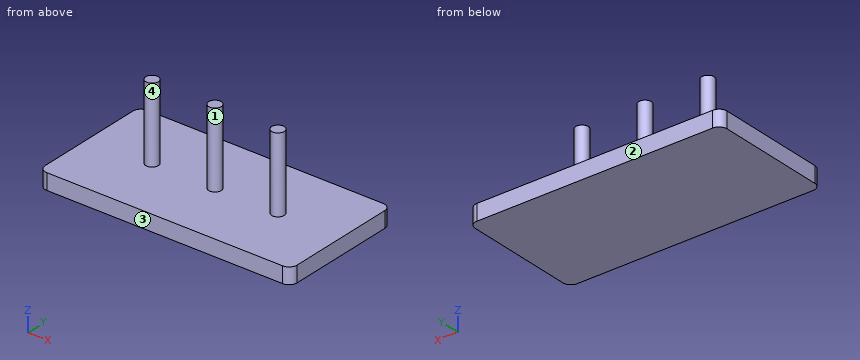
```python
from build123d import *

# Parameters (mm, degrees)
F0_W     = 400
F0_H     = 200
F1_DEPTH = 25.4
F2_R     = 10
F3_DEPTH = 120
F4_R     = 12.7


with BuildPart() as f1:
    # F0 (on Top) → F1 (new body)
    with BuildSketch(Plane.XY):
        Rectangle(F0_W, F0_H)
    extrude(amount=F1_DEPTH)

    # F2 (on face) → F3 (join)
    with BuildSketch(Plane.XY.offset(25.4)):
        Circle(F2_R)
        with Locations((100, 0)):
            Circle(F2_R)
        with Locations((-100, 0)):
            Circle(F2_R)
    extrude(amount=F3_DEPTH)

    # F4
    f4_edges = [f1.edges().sort_by_distance(p)[0] for p in [
        (200, -100, 12.7),
        (-200, -100, 12.7),
        (-200, 100, 12.7),
        (200, 100, 12.7),
    ]]
    fillet(f4_edges, radius=F4_R)


solid = f1.part
```
Work out the finished part from the listing and answer in its coordinate system (mm). Face numbers are marked on the shaded views. A direction names the side the tool comes from. Give positions to 0.01 mm unless a question says otherwise; leave off trailing zeros. Order: outer loops, then holes, each group sorted by start corner. A loop starts at its lowest first (then second) coordinate and runs counter-clockwise, first axis right, second up. Notation, with made-up numbers: M -11,45 L -5,45 A16 ccw -5,67 Z; hole C -25.75,89 d3. An arc over 180 degrees is marked long. Return JSON: item names as keys, results as strings.
1) Section D-D, the plane x = 62 is taken. Write down the section's boundary in (y, z), plus the area to 3 significant figures.
Resolved:
{"outline": "M -100,0 L 100,0 L 100,25.4 L -100,25.4 Z", "area": "5,080 mm^2"}
2) This flat-tipped pin is pushed along its axis until it touches: pin 1 (2 mm diameter, centred on x = -81.5, y = -56, fed in from +Z). Where does it stop, or does it pass through?
Resolved:
{"pin 1": "z = 25.4"}
3) Section C-C, the plane x = -100 is taken. Write down the section's boundary in (y, z), plus the area to 3 significant figures.
Resolved:
{"outline": "M -100,0 L 100,0 L 100,25.4 L 10,25.4 L 10,145.4 L -10,145.4 L -10,25.4 L -100,25.4 Z", "area": "7,480 mm^2"}
4) Straight lines are drawn through the part: line 1 along Z through (x, y) = (-171, -66); line 2 along X through (y, z) = (4, 28.5); line 3 along Y through (x, z) = (3, 39). For each, find the intervals that lie inside material, in ascending order. Write a range as [from, to].
Resolved:
{"line 1": "[0, 25.4]", "line 2": "[-109.17, -90.83], [-9.17, 9.17], [90.83, 109.17]", "line 3": "[-9.54, 9.54]"}
5) Section A-A, the plane z = 103 is taken. Write down the section's boundary in (x, y), plus the area to 3 significant figures.
Resolved:
{"outline": "C -100,0 d20; C 0,0 d20; C 100,0 d20", "area": "942 mm^2"}
6) A tool of negligible diameter and unlimited length cuts with its end or side. For the marked faces 3 and 4, from which of +Z, -Z, +X, -X, +Y, -Y can it reach the whole face along a straight path? Write none if from no direction.
Resolved:
{"face 3": "+Z, -Z, +X, -X, -Y", "face 4": "+Z"}
7) For a pull along X with two mould halves and no side action, classify the marked faces 1 and 2 as +X half, -X half, draft (parallel to the pull), parting line (faces both ways), or undercut.
Resolved:
{"face 1": "undercut", "face 2": "draft"}
8) Section B-B, the plane y = 0 is taken. Write down the section's boundary in (x, z), plus the area to 3 significant figures.
Resolved:
{"outline": "M -200,0 L 200,0 L 200,25.4 L 110,25.4 L 110,145.4 L 90,145.4 L 90,25.4 L 10,25.4 L 10,145.4 L -10,145.4 L -10,25.4 L -90,25.4 L -90,145.4 L -110,145.4 L -110,25.4 L -200,25.4 Z", "area": "17,400 mm^2"}
